Study the drawing (mm; zero at the part's minimum x, y, z) and answer. A direction names the side the tool comes from. Give positions to 0.01 mm unless a question says otherwise; leave off trailing zeros. Order: outer loops, then holes, each group sorted by start corner. A loop starts at its lowest first (then second) coordinate and runs counter-clockwise, first axis right, second up.
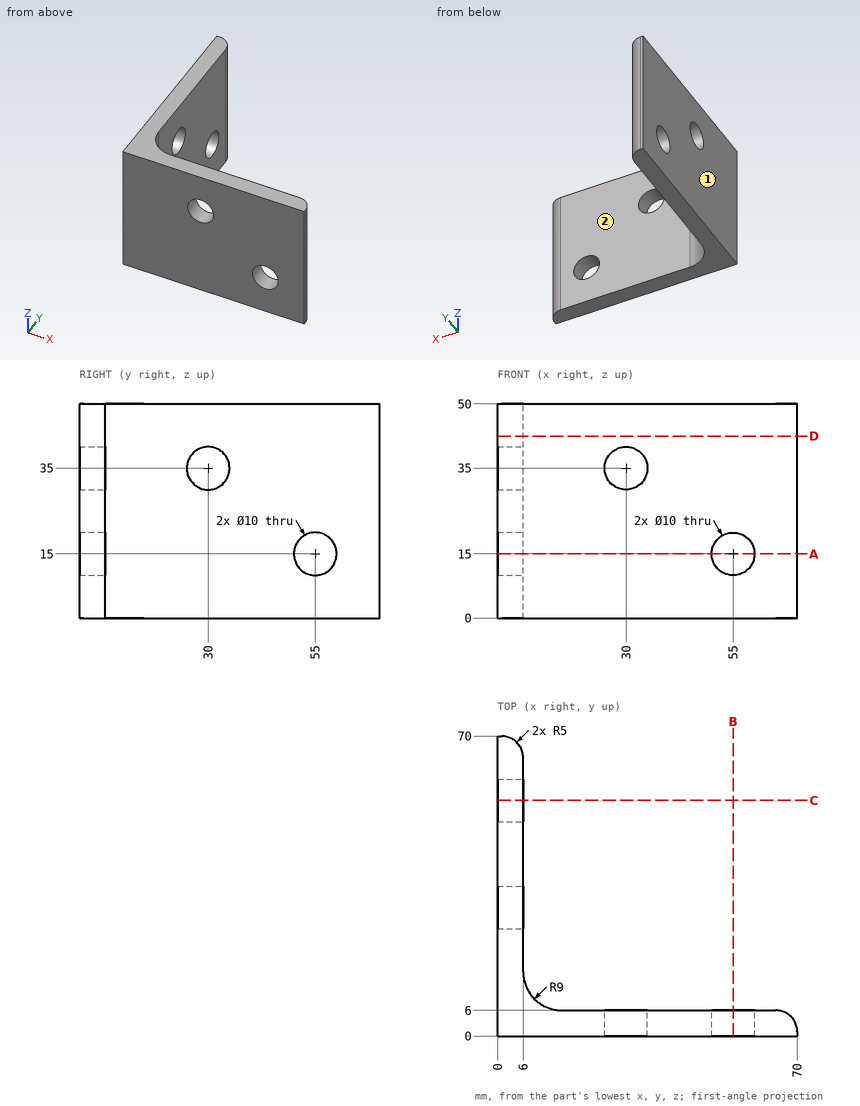
1) Find section D-D (z = 42.5). Write down the section's boundary in (x, y), then the cut area to 3 significant figures.
Geometry says:
outline: (0, 0) - (70, 0) - (70, 1) arc R5 ccw to (65, 6) - (15, 6) arc R9 cw to (6, 15) - (6, 65) arc R5 ccw to (1, 70) - (0, 70) - close
area: 811 mm2
2) Straight lines are drawn through the part: probe 1 along Y at (x, z) = (1, 15); probe 2 along Z at (x, y) = (1, 55); probe 3 along Y at (x, z) = (33, 7). For each, find the intervals that lie inside material, in ascending order.
Geometry says:
probe 1: y = 0 to 50, 60 to 70
probe 2: z = 0 to 10, 20 to 50
probe 3: y = 0 to 6
3) Find section A-A (z = 15). Write down the section's boundary in (x, y).
Geometry says:
outline: (0, 0) - (50, 0) - (50, 6) - (15, 6) arc R9 cw to (6, 15) - (6, 50) - (0, 50) - close; (0, 60) - (6, 60) - (6, 65) arc R5 ccw to (1, 70) - (0, 70) - close; (60, 0) - (70, 0) - (70, 1) arc R5 ccw to (65, 6) - (60, 6) - close
4) Find section B-B (x = 55). Write down the section's boundary in (y, z), then the cut area to 3 significant figures.
Geometry says:
outline: (0, 0) - (6, 0) - (6, 10) - (0, 10) - close; (0, 20) - (6, 20) - (6, 50) - (0, 50) - close
area: 240 mm2
5) A tool of negligible diameter and unlimited length cuts with its end or side. For the marked faces 1 and 2, from which of +Z, -Z, +X, -X, +Y, -Y can it reach the whole face along a straight path? Write none if from no direction.
Geometry says:
face 1: +Z, -Z, -X, +Y, -Y
face 2: +Z, -Z, +X, +Y
6) Given P1, Ø5, axis at x = 34, z = 9.5, coming from the +Y side; P2, Ø16, axis at y = 30, z = 35, coming from the +X side, each flat-ended and moving along its own axis, determine where each tip first touches the part or whether it passes through.
Geometry says:
P1: stops at y = 6
P2: stops at x = 6
